Check sheet for the modelled part. Datum: model origin and axes. Units: mm. A direction names the side the tool comes from. Give positions to 0.01 mm unless a question says otherwise; leave off trailing zeros. Write each loop counter-clockwise with the first axis right and the second up, starting at its lowest first coordinate (ties: lowest second). Pieces come first, ordered by that corner, then holes. Notation, with made-up numbers: M 49,58.25 L 107,58.25 A33 cw 107,97.25 Z; hole C 5,-7.5 d5. An arc over 180 degrees is marked long. Use CSV: the item, a comma, the result in double quotes. Start each with the question number.
1. Depth check by flat-ended pin: P1, Ø8, axis at x = -25.5, y = 11, coming from the -Z side; P2, Ø4, axis at y = -33, z = 28, coming from the -X side; P3, Ø12, axis at x = -9, z = 44.5, coming from the -Y side; P4, Ø1.5, axis at y = -32, z = 25.5, coming from the +X side. Enter the tip coordinate at first touch or a pass-through.
2. Cross-section at B-B, the plane y = 0. Enter the section's corners in (x, z).
3. Cross-section at A-A, the plane z = 21. Enter the section's corners in (x, y), and give its area (3 significant figures).
4. Cross-section at D-D, the plane z = 39.5. Enter the section's corners in (x, y), and give its area (3 significant figures).
5. Scan lines: line 1 (Y direction, x = 0, z = 53); line 2 (Y direction, x = 14.5, z = 31.5); line 3 (Z direction, x = 4, y = 22). Record each from-to range of solid material in increasing order.
6. Cross-section at C-C, the plane x = 20. Enter the section's corners in (y, z).
7. Access from +Z, -Z, +X, -X, +Y, -Y to the whole of each face (thin tool, end or side, straight path). Record for faces 1 (the face through (-2.17, -9.76, 57.4)), 2 (the face through (-5.269, -32.465, 16.042)), 3 (the face through (5.269, -32.465, 33.958)).
from build123d import *

# Parameters (mm, degrees)
F0_W     = 80
F0_H     = 60
F1_DEPTH = 50
F2_R     = 10
F3_DEPTH = 15
F5_DEPTH = 5


with BuildPart() as f1:
    # F0 (on Top) → F1 (new body)
    with BuildSketch(Plane.XY):
        Rectangle(F0_W, F0_H)
    extrude(amount=F1_DEPTH)

    # F2 (on face) → F3 (join)
    with BuildSketch(Plane.XY.offset(50)):
        Circle(F2_R)
    extrude(amount=F3_DEPTH)

    # F4 (on face) → F5 (join)
    with BuildSketch(Plane.XZ.offset(30)):
        Polygon((-10.392305, 19), (0, 13), (10.392305, 19), (10.392305, 31), (0, 37), (-10.392305, 31), align=None)
    extrude(amount=F5_DEPTH)


solid = f1.part
Worked answers:
1,P1,"stops at z = 0"
1,P2,"stops at x = -10.39"
1,P3,"stops at y = -30"
1,P4,"stops at x = 10.39"
2,outline,"M -40,0 L 40,0 L 40,50 L 10,50 L 10,65 L -10,65 L -10,50 L -40,50 Z"
3,outline,"M -40,-30 L -10.39,-30 L -10.39,-35 L 10.39,-35 L 10.39,-30 L 40,-30 L 40,30 L -40,30 Z"
3,area,"4,900 mm^2"
4,outline,"M -40,-30 L 40,-30 L 40,30 L -40,30 Z"
4,area,"4,800 mm^2"
5,line 1,"y = -10 to 10"
5,line 2,"y = -30 to 30"
5,line 3,"z = 0 to 50"
6,outline,"M -30,0 L 30,0 L 30,50 L -30,50 Z"
7,face 1,"+Z"
7,face 2,"-Z, -X, -Y"
7,face 3,"+Z, +X, -Y"
